from build123d import *

# Parameters (mm, degrees)
BOSS_EXTRUDE2_DEPTH = 5


with BuildPart() as part:
    # Sketch3 → Boss-Extrude2 (new body)
    with BuildSketch(Plane.XY):
        with BuildLine():
            ThreePointArc((-20.75, 8.312490601), (-26.3, 0), (-20.75, -8.312490601))
            Line((-20.75, -8.312490601), (-15.631666667, -10.436793755))
            ThreePointArc((-15.631666667, -10.436793755), (0, 0), (-15.631666667, 10.436793755))
            Line((-15.631666667, 10.436793755), (-20.75, 8.312490601))
        make_face()
        with BuildLine():
            Line((-15.882575695, -2), (-18.52, -2))
            Line((-18.52, -2), (-18.52, 2))
            Line((-18.52, 2), (-15.882575695, 2))
            ThreePointArc((-15.882575695, 2), (-6.3, 0), (-15.882575695, -2))
        make_face(mode=Mode.SUBTRACT)
    extrude(amount=BOSS_EXTRUDE2_DEPTH)


solid = part.part
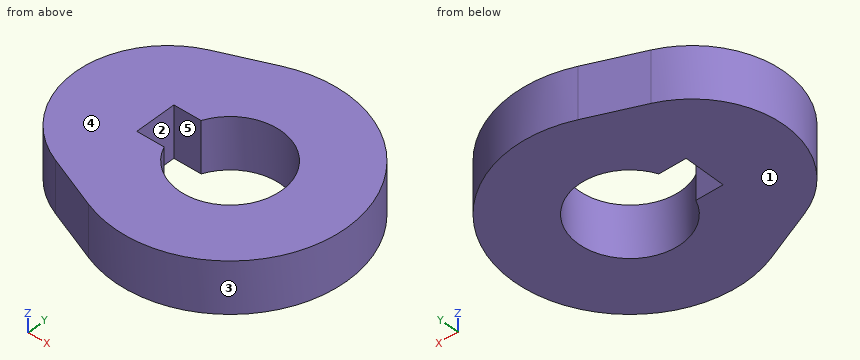
Verification items for the finished model (mm, model axes). Face numbers are marked on the shaded views. A direction names the side the tool comes from. Coordinates: 2 decimals unless noted, no trailing zeros. Write each loop counter-clockwise with the first axis right and the second up, starting at its lowest first coordinate (ties: lowest second). Pieces come first, ordered by that corner, then holes. Notation, with made-up numbers: (46.5, -38) - (99.5, -38) arc R20 ccw to (99.5, 0) - close; hole circle Ø10 at (-4.5, 34.5). An arc over 180 degrees is marked (long way). Answer as a JSON object with one key per item and string values.
(1) Gauge pin test, flat ends, axial feed: pin 1 Ø2 at (x, y) = (-15, -3) entering from -Z; pin 2 Ø0.8 at (x, z) = (-17.5, 2.5) entering from -Y; pin 3 Ø8 at (x, y) = (-11.3, 0) entering from -Z; pin 4 Ø1.3 at (x, z) = (-16.5, 1.5) entering from +Y. Record the tip position at first contact, or that the pin passes through.
Report:
{"pin 1": "z = 0", "pin 2": "y = -9.83", "pin 3": "through", "pin 4": "y = 10.35"}
(2) Tool access check on the marked faces 4 and 5. Record the directions out of +Z, -Z, +X, -X, +Y, -Y that give a thin tool (end or side, any length) a straight path to the whole face; none if there is none.
Report:
{"face 4": "+Z, +X, -X, +Y, -Y", "face 5": "+Z, -Z"}
(3) Mould release check, pull along X, two halves, no side actions. Record for the marked faces 1, 2 and 3: pulls with the +X half, pulls with the -X half, needs draft (parallel to the pull), parting line crosses it, or undercut.
Report:
{"face 1": "needs draft", "face 2": "undercut", "face 3": "parting line crosses it"}
(4) Cross-section at A-A on x = -11.3. Record the cut outline in (y, z), plus the area to 3 significant figures.
Report:
{"outline": "(-11.3, 0) - (-5, 0) - (-5, 5) - (-11.3, 5) - close; (5, 0) - (11.3, 0) - (11.3, 5) - (5, 5) - close", "area": "63.0 mm^2"}
(5) Cross-section at D-D on x = -24.25. Record the cut outline in (y, z).
Report:
{"outline": "(-5.72, 0) - (5.72, 0) - (5.72, 5) - (-5.72, 5) - close"}
(6) Cross-section at B-B on z = 4.45. Record the cut outline in (x, y), plus the area to 3 significant figures.
Report:
{"outline": "(-20.75, -8.31) - (-15.63, -10.44) arc R11.3 ccw (long way) to (-15.63, 10.44) - (-20.75, 8.31) arc R9 ccw to start; hole (-18.52, -2) - (-15.88, -2) arc R5 ccw (long way) to (-15.88, 2) - (-18.52, 2) - close", "area": "371 mm^2"}
(7) Cross-section at C-C on y = 0. Record the cut outline in (x, z).
Report:
{"outline": "(-26.3, 0) - (-18.52, 0) - (-18.52, 5) - (-26.3, 5) - close; (-6.3, 0) - (0, 0) - (0, 5) - (-6.3, 5) - close"}
(8) Thickness scan on line 1 along X through (y, z) = (0, 1.9); line 2 along Y through (x, z) = (-11.3, 3.45); line 3 along X through (y, z) = (4, 2.7). Record the ranges inside material, lowest first.
Report:
{"line 1": "-26.3 to -18.52, -6.3 to 0", "line 2": "-11.3 to -5, 5 to 11.3", "line 3": "-25.36 to -14.3, -8.3 to -0.73"}
